For this review, take the finished solid that the model builds, in its own axes (mm). Coordinates: 2 decimals unless noted, no trailing zeros. Loops run counter-clockwise (first coordinate to the right, second up) from the corner with the lowest first, then second, coordinate; pieces in that order, holes last.
1. Take a section at B-B, the plane z = 2.45. Count the separate pieces of the cut face and the enclosed holes in it, then the cut area to 3 significant figures.
2. Clearance check with flat-ended pins moving along their axes: P1, Ø1.5, axis at x = 107.53, y = 5, coming from the -Z side; P2, Ø1, axis at y = -2.5, z = 2, coming from the +X side; P3, Ø1, axis at x = 129, z = 1.5, coming from the +Y side. State where each tip first meets the part, or that it passes through.
3. Take a section at C-C, the plane x = 144.5. State the section outline as (y, z) points, then the cut area to 3 significant figures.
4. Take a section at A-A, the plane y = 5. State the section outline as (x, z) points.
5. Mouldability with a two-part tool opening along Y and no side actions: class faces 1 (the face through (124, 5, 0)), 2 (the face through (152.47, -6.49, 1.48)), 3 (the face through (108.64, 5.58, 1.48)) as pulls with the +Y half, pulls with the -Y half, needs draft (parallel to the pull), parting line crosses it, or undercut.
6. Take a section at D-D, the plane x = 111.5. State the section outline as (y, z) points.
7. To check wall thickness, follow probe 1 along Y at (x, z) = (150, 0.2); probe 2 along Y at (x, z) = (101, 1); probe 3 along Y at (x, z) = (103.5, 0.5). State the ranges of each line that lie inside material, in increasing order.
```python
from build123d import *

# Parameters (mm, degrees)
SKETCH1_R           = 30
BOSS_EXTRUDE1_DEPTH = 3
LPATTERN1_COUNT     = 2
LPATTERN1_PITCH     = 8
CIRPATTERN1_COUNT   = 4


with BuildPart() as part:
    # Sketch1 → Boss-Extrude1 (new body)
    with BuildSketch(Plane.XY):
        with Locations((124.757462076, 5)):
            Circle(SKETCH1_R)
    extrude(amount=BOSS_EXTRUDE1_DEPTH)

    # Sketch2 → M3 Tapped Hole1 (revolve, cut)
    with BuildSketch(Plane(origin=(107.532834786, 5, 0), x_dir=(0, 1, 0), z_dir=(1, 0, 0))):
        Polygon((0, 0), (0, 8.251075774), (1.25, 7.5), (1.25, 0), align=None)
    m3_tapped_hole1 = revolve(axis=Axis((107.532834786, 5, -6.35), (0, 0, 1)), mode=Mode.SUBTRACT)

    # LPattern1: M3 Tapped Hole1 ×2
    with Locations(*[(-i * LPATTERN1_PITCH, 0, 0) for i in range(1, LPATTERN1_COUNT)]):
        add(m3_tapped_hole1, mode=Mode.SUBTRACT)

    # CirPattern1: M3 Tapped Hole1 ×4 about axis
    cirpattern1_axis = Axis((124.757462076, 5, 0), (0, 0, 1))
    for i in range(1, CIRPATTERN1_COUNT):
        add(m3_tapped_hole1.rotate(cirpattern1_axis, i * 360 / CIRPATTERN1_COUNT), mode=Mode.SUBTRACT)

    # CirPattern1 copy 1 sketch → CirPattern1 copy 1 (revolve, cut)
    with BuildSketch(Plane(origin=(124.757462076, -20.22462729, 0), x_dir=(-1, 0, 0), z_dir=(0, 1, 0))):
        Polygon((0, 0), (0, 8.251075774), (1.25, 7.5), (1.25, 0), align=None)
    revolve(axis=Axis((124.757462076, -20.22462729, -6.35), (0, 0, 1)), mode=Mode.SUBTRACT)

    # CirPattern1 copy 2 sketch → CirPattern1 copy 2 (revolve, cut)
    with BuildSketch(Plane(origin=(149.982089365, 5, 0), x_dir=(0, -1, 0), z_dir=(-1, 0, 0))):
        Polygon((0, 0), (0, 8.251075774), (1.25, 7.5), (1.25, 0), align=None)
    revolve(axis=Axis((149.982089365, 5, -6.35), (0, 0, 1)), mode=Mode.SUBTRACT)

    # CirPattern1 copy 3 sketch → CirPattern1 copy 3 (revolve, cut)
    with BuildSketch(Plane(origin=(124.757462076, 30.22462729, 0), x_dir=(1, 0, 0), z_dir=(0, -1, 0))):
        Polygon((0, 0), (0, 8.251075774), (1.25, 7.5), (1.25, 0), align=None)
    revolve(axis=Axis((124.757462076, 30.22462729, -6.35), (0, 0, 1)), mode=Mode.SUBTRACT)


solid = part.part
```
Results list:
1. separate pieces: 1
1. enclosed holes: 8
1. area: 2,790 mm2
2. P1: passes through
2. P2: stops at x = 153.93
2. P3: stops at y = 34.77
3. outline: (-17.59, 0) - (27.59, 0) - (27.59, 3) - (-17.59, 3) - close
3. area: 136 mm2
4. outline: (94.76, 0) - (98.28, 0) - (98.28, 3) - (94.76, 3) - close; (100.78, 0) - (106.28, 0) - (106.28, 3) - (100.78, 3) - close; (108.78, 0) - (140.73, 0) - (140.73, 3) - (108.78, 3) - close; (143.23, 0) - (148.73, 0) - (148.73, 3) - (143.23, 3) - close; (151.23, 0) - (154.76, 0) - (154.76, 3) - (151.23, 3) - close
5. face 1: needs draft
5. face 2: parting line crosses it
5. face 3: undercut
6. outline: (-21.91, 0) - (31.91, 0) - (31.91, 3) - (-21.91, 3) - close
7. probe 1: y = -11.21 to 3.75, 6.25 to 21.21
7. probe 2: y = -13.32 to 23.32
7. probe 3: y = -16.17 to 26.17
